Can you work these out from the model? Positions are in its coordinate system, mm. A direction names the side the tool comes from. Round coordinates to 2 decimals unless told otherwise and drop trailing zeros. Write each loop counter-clockwise with the first axis right and the second up, starting at its lowest first coordinate (ties: lowest second). Pieces come first, ordered by that corner, then holes.
Q1. If we section it at D-D (y = 8.5): Please give me the cut outline in (x, z), plus the area to 3 significant figures.
Q2. We'd pull the mould along X, two halves only. Please class faces 1 (the flat face through (23, 3, -14.662)), 2 (the flat face through (0, 1, -13)): +X half, -X half, draft (parallel to the pull), parting line (faces both ways), or undercut.
Q3. If we section it at A-A (y = 2.25): Please give me the cut outline in (x, z), plus the area to 4 significant figures.
Q4. Please list where these lines run through material, in increasing order: line 1 along X through (y, z) = (8.25, -22.75); line 2 along Z through (x, y) = (39.5, 9.5); line 3 along X through (y, z) = (13.5, -12.5).
Q5. If we section it at C-C (x = 27): Please give me the cut outline in (y, z).
Q6. I'm going to push flat-ended pins straight in: pin 1 Ø2.5 at (y, z) = (9.5, -23) entering from -X; pin 2 Ø5 at (x, z) = (50, -22) entering from -Y; pin 3 Ø1 at (y, z) = (4.5, -7.5) entering from -X; pin 4 Ø4 at (x, y) = (4, 10.5) entering from +Z. Where does each tip first touch, or does it pass through?
Q7. For faces 3 (the flat face through (57, 8, -14.922)), 4 (the flat face through (9.43, 8, -17)), 5 (the flat face through (23, 4.59, -19)), 6 (the flat face through (57, 8, -4.906)), which set-ups out of +Z, -Z, +X, -X, +Y, -Y let a thin tool reach every point of the face, with its end or its side?
Q8. If we section it at B-B (z = -15.5): Please give me the cut outline in (x, y), plus the area to 3 significant figures.
from build123d import *

# Parameters (mm, degrees)
SKETCH1_W           = 61.7
SKETCH1_H           = 26.2
BOSS_EXTRUDE1_DEPTH = 1.59
SKETCH2_R           = 4.284216932
SKETCH2_R_2         = 4.233461823
SKETCH2_W           = 7.996291091
SKETCH2_H           = 11.231630152
SKETCH2_W_2         = 6.79740416
SKETCH2_H_2         = 10.015433833
SKETCH2_W_3         = 3.744475554
SKETCH2_H_3         = 8.537740598
SKETCH2_W_4         = 3.804793914
BOSS_EXTRUDE2_DEPTH = 13
FILLET1_R           = 1
SKETCH3_W           = 11.824805187
SKETCH3_H           = 9.14941117
BOSS_EXTRUDE3_DEPTH = 3


with BuildPart() as part:
    # Sketch1 → Boss-Extrude1 (new body)
    with BuildSketch(Plane(origin=(0, 0, 0), x_dir=(1, 0, 0), z_dir=(0, 1, 0))):
        with Locations((30.85, 13.1)):
            Rectangle(SKETCH1_W, SKETCH1_H)
    extrude(amount=BOSS_EXTRUDE1_DEPTH)

    # Sketch2 → Boss-Extrude2 (add)
    with BuildSketch(Plane(origin=(0, 1.59, 0), x_dir=(1, 0, 0), z_dir=(0, 1, 0))):
        with Locations((50.601195051, 21.255565251)):
            Circle(SKETCH2_R)
        with Locations((12.398624263, 6.095655225)):
            Circle(SKETCH2_R_2)
        with Locations((5.431373533, 16.986694952)):
            Rectangle(SKETCH2_W, SKETCH2_H)
        with Locations((56.574526606, 9.914115999)):
            Rectangle(SKETCH2_W_2, SKETCH2_H_2)
        with Locations((36.301503569, 21.255565251)):
            Rectangle(SKETCH2_W_3, SKETCH2_H_3)
        with Locations((41.260345926, 21.255565251)):
            Rectangle(SKETCH2_W_4, SKETCH2_H_3)
    extrude(amount=BOSS_EXTRUDE2_DEPTH)

    # Fillet1
    fillet1_edges = [part.edges().sort_by_distance(p)[0] for p in [
        (46.316978119, 14.59, -21.255565251),
        (8.16516244, 14.59, -6.095655225),
    ]]
    fillet(fillet1_edges, radius=FILLET1_R)

    # Sketch3 → Boss-Extrude3 (add)
    with BuildSketch(Plane(origin=(0, 1.59, 0), x_dir=(1, 0, 0), z_dir=(0, 1, 0))):
        with Locations((22.821277789, 19.236524015)):
            Rectangle(SKETCH3_W, SKETCH3_H)
    extrude(amount=BOSS_EXTRUDE3_DEPTH)


solid = part.part
A:
1. outline: (1.43, -22.6) - (9.43, -22.6) - (9.43, -11.37) - (1.43, -11.37) - close; circle Ø8.47 at (12.4, -6.1); (34.43, -25.52) - (38.17, -25.52) - (38.17, -16.99) - (34.43, -16.99) - close; (39.36, -25.52) - (43.16, -25.52) - (43.16, -16.99) - (39.36, -16.99) - close; circle Ø8.57 at (50.6, -21.26); (53.18, -14.92) - (59.97, -14.92) - (59.97, -4.91) - (53.18, -4.91) - close
1. area: 336 mm2
2. face 1: undercut
2. face 2: -X half
3. outline: (1.43, -22.6) - (9.43, -22.6) - (9.43, -11.37) - (1.43, -11.37) - close; circle Ø8.47 at (12.4, -6.1); (16.91, -23.81) - (28.73, -23.81) - (28.73, -14.66) - (16.91, -14.66) - close; (34.43, -25.52) - (38.17, -25.52) - (38.17, -16.99) - (34.43, -16.99) - close; (39.36, -25.52) - (43.16, -25.52) - (43.16, -16.99) - (39.36, -16.99) - close; circle Ø8.57 at (50.6, -21.26); (53.18, -14.92) - (59.97, -14.92) - (59.97, -4.91) - (53.18, -4.91) - close
3. area: 444.5 mm2
4. line 1: x = 34.43 to 38.17, 39.36 to 43.16, 46.59 to 54.62
4. line 2: z = -25.52 to -16.99
4. line 3: x = 1.43 to 9.43, 53.18 to 59.97
5. outline: (0, -26.2) - (1.59, -26.2) - (1.59, -23.81) - (4.59, -23.81) - (4.59, -14.66) - (1.59, -14.66) - (1.59, 0) - (0, 0) - close
6. pin 1: stops at x = 1.43
6. pin 2: stops at y = 0
6. pin 3: stops at x = 8.26
6. pin 4: stops at z = -11.37
7. face 3: +X, +Y
7. face 4: -Z, +Y
7. face 5: +Z, -Z, +Y
7. face 6: +Z, +X, +Y
8. outline: (0, 0) - (61.7, 0) - (61.7, 1.59) - (28.73, 1.59) - (28.73, 4.59) - (16.91, 4.59) - (16.91, 1.59) - (9.43, 1.59) - (9.43, 14.59) - (1.43, 14.59) - (1.43, 1.59) - (0, 1.59) - close
8. area: 238 mm2
